from build123d import *

# Parameters (mm, degrees)
SKETCH_1_W              = 75.71
SKETCH_1_H              = 32
SKETCH_1_R              = 1.6
EXTRUDE_1_DEPTH         = 3
SHEET_START             = -1
SHEET_METAL_1_OUTLINE_W = 75.71
SHEET_METAL_1_OUTLINE_H = 32
SHEET_METAL_1_OUTLINE_R = 1.6
SHEET_METAL_1_DEPTH     = 1
SM_EDGE_FLANGE_1_DEPTH  = 75.71
SKETCH_26_R             = 4.05
SKETCH_26_R_2           = 1.6
CUT_EXTRUDE_1_DEPTH     = 10
FILLET_4_R              = 3
M4X0_7_1_D              = 3.3


# Read off the part's stored shape, not the designer's step: 轉換-實體1
# Sheet-metal steps are written as plain solids
with BuildPart() as part:
    # Sketch 1 → 填料-伸長1 (new body)
    with BuildSketch(Plane.XY):
        with Locations((37.855, -16)):
            Rectangle(SKETCH_1_W, SKETCH_1_H)
        with Locations((36, -5)):
            Circle(SKETCH_1_R, mode=Mode.SUBTRACT)
        with Locations((16, -5)):
            Circle(SKETCH_1_R, mode=Mode.SUBTRACT)
        with Locations((16, -25)):
            Circle(SKETCH_1_R, mode=Mode.SUBTRACT)
        with Locations((36, -25)):
            Circle(SKETCH_1_R, mode=Mode.SUBTRACT)
    extrude(amount=EXTRUDE_1_DEPTH)

    # Sheet Metal 1 outline → Sheet Metal 1 (add)
    with BuildSketch(Plane.XY.offset(SHEET_START)):
        with Locations((37.855, -16)):
            Rectangle(SHEET_METAL_1_OUTLINE_W, SHEET_METAL_1_OUTLINE_H)
        with Locations((16, -25)):
            Circle(SHEET_METAL_1_OUTLINE_R, mode=Mode.SUBTRACT)
        with Locations((36, -25)):
            Circle(SHEET_METAL_1_OUTLINE_R, mode=Mode.SUBTRACT)
        with Locations((16, -5)):
            Circle(SHEET_METAL_1_OUTLINE_R, mode=Mode.SUBTRACT)
        with Locations((36, -5)):
            Circle(SHEET_METAL_1_OUTLINE_R, mode=Mode.SUBTRACT)
    extrude(amount=SHEET_METAL_1_DEPTH)

    # 邊線-凸緣1 section (across the edge) → 邊線-凸緣1 (add)
    with BuildSketch(Plane(origin=(75.71, 2, 3), x_dir=(0, -1, 0), z_dir=(-1, 0, 0))):
        with BuildLine():
            Line((-4, 2), (-4, 66))
            Line((-4, 66), (0, 66))
            Line((0, 66), (0, 2))
            ThreePointArc((0, 2), (0.585786438, 0.585786438), (2, 0))
            Line((2, 0), (2, -4))
            ThreePointArc((2, -4), (-2.242640687, -2.242640687), (-4, 2))
        make_face()
    extrude(amount=SM_EDGE_FLANGE_1_DEPTH)

    # 草圖26 → 除料-伸長1 (cut)
    with BuildSketch(Plane(origin=(0, 6, 0), x_dir=(1, 0, 0), z_dir=(0, 1, 0))):
        with Locations(Location((36.28, -59, 0), (0, 0, 270))):
            Circle(SKETCH_26_R)
        with Locations(Location((15, -9.05, 0), (0, 0, 270))):
            Circle(SKETCH_26_R_2)
        with Locations(Location((25, -9.05, 0), (0, 0, 270))):
            Circle(SKETCH_26_R_2)
        with Locations(Location((15, -29.05, 0), (0, 0, 270))):
            Circle(SKETCH_26_R_2)
        with Locations(Location((25, -29.05, 0), (0, 0, 270))):
            Circle(SKETCH_26_R_2)
    extrude(amount=-CUT_EXTRUDE_1_DEPTH, mode=Mode.SUBTRACT)

    # 圓角4
    fillet_4_edges = [part.edges().sort_by_distance(p)[0] for p in [
        (0, -32, 1),
        (75.71, -32, 1),
        (75.71, 4, 69),
        (0, 4, 69),
    ]]
    fillet(fillet_4_edges, radius=FILLET_4_R)

    # M4x0.7 螺紋孔1 (through all)
    with Locations(Plane(origin=(70.71, 6, 54), x_dir=(0, 0, 1), z_dir=(0, 1, 0))):
        with Locations((0, 0), (10, 0), (10, -49.5), (0, -49.5)):
            Hole(M4X0_7_1_D / 2)


solid = part.part
Could you check a few things on this model? Use its own coordinates, in mm. A direction names the side the tool comes from. Give positions to 0.01 mm unless a question says otherwise; leave off trailing zeros. Order: outer loops, then holes, each group sorted by start corner. A loop starts at its lowest first (then second) coordinate and runs counter-clockwise, first axis right, second up. Notation, with made-up numbers: (17.25, 71.25) -> (49.25, 71.25) arc R17 ccw to (49.25, 83.25) -> close; hole circle Ø2 at (-40, 44.5). An arc over 180 degrees is marked (long way). Answer in a Markdown table with one row per item. Add a question column.
Item 1: Imagine slicing it at A-A (z = 54). List the corners of the cut face in (x, y) for me, and give its area (3 significant figures).
Item 2: Imagine slicing it at B-B (y = -5). List the corners of the cut face in (x, z) for me.
Item 3: I'm going to push flat-ended pins straight in: P1, Ø19, axis at x = 44.5, z = 22, coming from the -Y side; P2, Ø4, axis at x = 47.5, y = -1.5, coming from the +Z side; P3, Ø8, axis at x = 59.5, y = -11.5, coming from the +Z side. Where does each tip first touch, or does it pass through?
Item 4: For faces 5 (the flat face through (38, 4, 69)), 6 (the flat face through (37, -16, 3)), which set-ups out of +Z, -Z, +X, -X, +Y, -Y let a thin tool reach every point of the face, with its end or its side?
Item 5: We'd pull the mould along Y, two halves only. Please class faces 1 (the cylindrical face through (15.481, 4.028, 30.576)), 2 (the cylindrical face through (34.82, -23.92, 0.97)), 3 (the cylindrical face through (74.85, -31.1, 1.03)), 4 (the cylindrical face through (14.4, -24.93, 0.97)): pulls with the +Y half, pulls with the -Y half, needs draft (parallel to the pull), parting line crosses it, or undercut.
Item 6: Imagine slicing it at C-C (x = 21.21). List the corners of the cut face in (y, z) for me, and give its area (3 significant figures).
Item 7: Please list where these lines run through material, in increasing order: probe 1 along Y at (x, z) = (16, -0.2); probe 2 along X at (y, z) = (4.2, 9.05); probe 3 along X at (y, z) = (3, 54).
Item 8: Imagine slicing it at D-D (x = 49.5). List the corners of the cut face in (y, z) for me, and give its area (3 significant figures).
Result:
| question | item | result |
|---|---|---|
| 1 | outline | (0, 2) -> (19.56, 2) -> (19.56, 6) -> (0, 6) -> close; (22.86, 2) -> (69.06, 2) -> (69.06, 6) -> (22.86, 6) -> close; (72.36, 2) -> (75.71, 2) -> (75.71, 6) -> (72.36, 6) -> close |
| 1 | area | 276 mm2 |
| 2 | outline | (0, -1) -> (14.4, -1) -> (14.4, 3) -> (0, 3) -> close; (17.6, -1) -> (34.4, -1) -> (34.4, 3) -> (17.6, 3) -> close; (37.6, -1) -> (75.71, -1) -> (75.71, 3) -> (37.6, 3) -> close |
| 3 | P1 | y = 2 |
| 3 | P2 | z = 3.06 |
| 3 | P3 | z = 3 |
| 4 | face 5 | +Z, +X, -X, +Y, -Y |
| 4 | face 6 | +Z, +X, -X, -Y |
| 5 | face 1 | needs draft |
| 5 | face 2 | undercut |
| 5 | face 3 | pulls with the -Y half |
| 5 | face 4 | undercut |
| 6 | outline | (-32, -1) -> (0, -1) arc R6 ccw to (6, 5) -> (6, 52.35) -> (2, 52.35) -> (2, 5) arc R2 cw to (0, 3) -> (-32, 3) -> close; (2, 55.65) -> (6, 55.65) -> (6, 62.35) -> (2, 62.35) -> close; (2, 65.65) -> (6, 65.65) -> (6, 69) -> (2, 69) -> close |
| 6 | area | 383 mm2 |
| 7 | probe 1 | -32 to -26.6, -23.4 to -6.6, -3.4 to 2.99 |
| 7 | probe 2 | 0 to 13.4, 16.6 to 23.4, 26.6 to 75.71 |
| 7 | probe 3 | 0 to 19.56, 22.86 to 69.06, 72.36 to 75.71 |
| 8 | outline | (-32, -1) -> (0, -1) arc R6 ccw to (6, 5) -> (6, 69) -> (2, 69) -> (2, 5) arc R2 cw to (0, 3) -> (-32, 3) -> close |
| 8 | area | 409 mm2 |
